Part model, mm, in its own coordinate system. Round coordinates to 2 decimals unless told otherwise and drop trailing zeros. Loops run counter-clockwise (first coordinate to the right, second up) from the corner with the lowest first, then second, coordinate; pieces in that order, holes last. Notation, with made-up numbers: (36, 61) - (83, 61) arc R19 cw to (83, 98) - close; hole circle Ø4 at (89, 21.25). An arc over 180 degrees is marked (long way). Write each question's results on one line, items separated by ' | '. Start each with the question number.
(1) Cut at B-B, the plane y = 0. List the corners of the cut face in (x, z), then the cut area to 3 significant figures.
(2) Cut at C-C, the plane x = 0.75. List the corners of the cut face in (y, z).
(3) Flat gauge pins, fed straight in: P1, Ø0.9, axis at x = -0.5, z = -6, coming from the -Y side; P2, Ø1.5, axis at x = -0.5, z = -17, coming from the +Y side. Where does each tip first touch, or does it go through?
(4) Drill centre lines: L1, parallel to Y at x = 0.7, z = -62.5; L2, parallel to Z at x = 0.45, y = -0.75; L3, parallel to Z at x = -0.6, y = 0.5. Where is each one in solid material? Low to high.
(5) Cut at D-D, the plane z = 41. List the corners of the cut face in (x, y), then the cut area to 3 significant figures.
(6) Cut at A-A, the plane z = -62.5. List the corners of the cut face in (x, y).
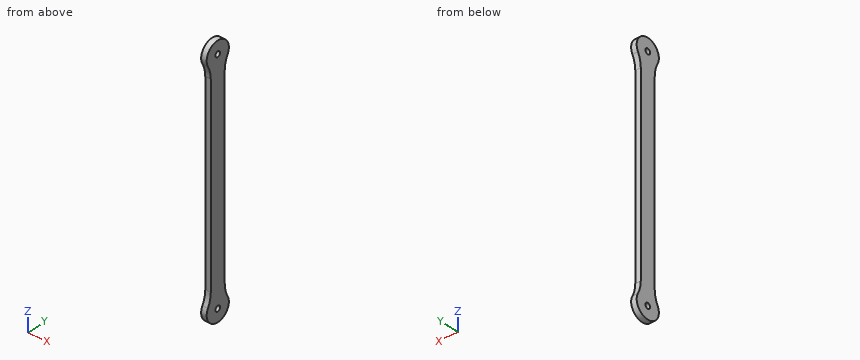
from build123d import *

# Parameters (mm, degrees)
SKETCH1_R           = 6.75
SKETCH1_R_2         = 1.45
BOSS_EXTRUDE1_DEPTH = 1.5
FILLET1_R           = 15


with BuildPart() as part:
    # Sketch1 → Boss-Extrude1 (new body, symmetric)
    with BuildSketch(Plane(origin=(0, 0, 0), x_dir=(0, 0, -1), z_dir=(1, 0, 0))):
        with Locations((-62.5, 0)):
            Circle(SKETCH1_R)
        with Locations((-62.5, 0)):
            Circle(SKETCH1_R_2, mode=Mode.SUBTRACT)
        with BuildLine():
            Line((-57.255955759, -4.25), (57.255955759, -4.25))
            ThreePointArc((57.255955759, -4.25), (55.75, 0), (57.255955759, 4.25))
            Line((57.255955759, 4.25), (-57.255955759, 4.25))
            ThreePointArc((-57.255955759, 4.25), (-56.137618424, 2.254462394), (-55.75, 0))
            ThreePointArc((-55.75, 0), (-56.137618424, -2.254462394), (-57.255955759, -4.25))
        make_face()
        with Locations((62.5, 0)):
            Circle(SKETCH1_R)
        with Locations((62.5, 0)):
            Circle(SKETCH1_R_2, mode=Mode.SUBTRACT)
    extrude(amount=BOSS_EXTRUDE1_DEPTH, both=True)

    # Fillet1
    fillet1_edges = [part.edges().sort_by_distance(p)[0] for p in [
        (0, 4.25, -57.255955759),
        (0, -4.25, -57.255955759),
        (0, -4.25, 57.255955759),
        (0, 4.25, 57.255955759),
    ]]
    fillet(fillet1_edges, radius=FILLET1_R)


solid = part.part
A:
1) outline: (-1.5, -69.25) - (1.5, -69.25) - (1.5, -63.95) - (-1.5, -63.95) - close; (-1.5, -61.05) - (1.5, -61.05) - (1.5, 61.05) - (-1.5, 61.05) - close; (-1.5, 63.95) - (1.5, 63.95) - (1.5, 69.25) - (-1.5, 69.25) - close | area: 398 mm2
2) outline: (-5.97, -59.36) arc R6.75 ccw (long way) to (5.97, -59.36) arc R15 cw to (4.25, -52.38) - (4.25, 52.38) arc R15 cw to (5.97, 59.36) arc R6.75 ccw (long way) to (-5.97, 59.36) arc R15 cw to (-4.25, 52.38) - (-4.25, -52.38) arc R15 cw to start; hole circle Ø2.9 at (0, -62.5); hole circle Ø2.9 at (0, 62.5)
3) P1: y = -4.25 | P2: y = 4.25
4) L1: -6.75 to -1.45, 1.45 to 6.75 | L2: -69.21 to -63.74, -61.26 to 61.26, 63.74 to 69.21 | L3: -69.23 to -63.86, -61.14 to 61.14, 63.86 to 69.23
5) outline: (-1.5, -4.25) - (1.5, -4.25) - (1.5, 4.25) - (-1.5, 4.25) - close | area: 25.5 mm2
6) outline: (-1.5, -6.75) - (1.5, -6.75) - (1.5, -1.45) - (-1.5, -1.45) - close; (-1.5, 1.45) - (1.5, 1.45) - (1.5, 6.75) - (-1.5, 6.75) - close
